Verification items for the finished model (mm, model axes). A direction names the side the tool comes from. Round coordinates to 2 decimals unless told otherwise and drop trailing zeros. Loops run counter-clockwise (first coordinate to the right, second up) from the corner with the lowest first, then second, coordinate; pieces in that order, holes last. Notation, with made-up numbers: M 0,17 L 31,17 A11 cw 31,25 Z; hole C 43.5,42 d4. An arc over 180 degrees is marked long. One line per item, written item: value.
from build123d import *

# Parameters (mm, degrees)
F0_W     = 50
F0_H     = 140
F1_DEPTH = 3
F3_D     = 5
F5_DEPTH = 39.832257


with BuildPart() as f1:
    # F0 (on Top) → F1 (new body)
    with BuildSketch(Plane.XY):
        with Locations((25, 70)):
            Rectangle(F0_W, F0_H)
    extrude(amount=-F1_DEPTH)

    # F3 (through all)
    with Locations(Plane.XY):
        with Locations((30, 86), (30, 62)):
            Hole(F3_D / 2)

    # F4 (on face) → F5 (cut)
    with BuildSketch(Plane.XY):
        with BuildLine():
            ThreePointArc((40.989516, 50), (43.489516, 47.5), (45.989516, 50))
            Line((45.989516, 50), (45.989516, 98))
            ThreePointArc((45.989516, 98), (43.489516, 100.5), (40.989516, 98))
            Line((40.989516, 98), (40.989516, 50))
        make_face()
    extrude(amount=-F5_DEPTH, mode=Mode.SUBTRACT)

    # F6: F1 across plane


with BuildPart() as f1_1:
    add(f1.part)
    add(f1.part.mirror(Plane.YZ))


solid = f1_1.part
(1) Sectioned sample at A-A on x = -30. Enter the section's corners in (y, z).
Completed:
outline: M 0,-3 L 59.5,-3 L 59.5,0 L 0,0 Z; M 64.5,-3 L 83.5,-3 L 83.5,0 L 64.5,0 Z; M 88.5,-3 L 140,-3 L 140,0 L 88.5,0 Z
(2) Sectioned sample at C-C on z = -1.25. Enter the section's corners in (x, y), and give its area (3 significant figures).
Completed:
outline: M -50,0 L 50,0 L 50,140 L -50,140 Z; hole M -45.99,50 A2.5 ccw -40.99,50 L -40.99,98 A2.5 ccw -45.99,98 Z; hole C -30,62 d5; hole C -30,86 d5; hole C 30,62 d5; hole C 30,86 d5; hole M 40.99,50 A2.5 ccw 45.99,50 L 45.99,98 A2.5 ccw 40.99,98 Z
area: 13,400 mm^2
(3) Sectioned sample at B-B on y = 86. Enter the section's corners in (x, z), and give its area (3 significant figures).
Completed:
outline: M -50,-3 L -45.99,-3 L -45.99,0 L -50,0 Z; M -40.99,-3 L -32.5,-3 L -32.5,0 L -40.99,0 Z; M -27.5,-3 L 27.5,-3 L 27.5,0 L -27.5,0 Z; M 32.5,-3 L 40.99,-3 L 40.99,0 L 32.5,0 Z; M 45.99,-3 L 50,-3 L 50,0 L 45.99,0 Z
area: 240 mm^2
(4) Mould release check, pull along X, two halves, no side actions. Record for faces 1 (the face through (1, 0, -1)), 2 (the face through (-50, 69, -1)), 3 (the face through (-43.5, 100.5, -1.5)): +X half, -X half, draft (parallel to the pull), parting line (faces both ways), or undercut.
Completed:
face 1: draft
face 2: -X half
face 3: undercut
(5) Thickness scan on L1, parallel to Y at x = 30, z = -1.7; L2, parallel to X at y = 55.5, z = -0.3; L3, parallel to X at y = 98.5, z = -2.05. Record the ranges inside material, lowest first. Write a range as from..to.
Completed:
L1: y = 0..59.5, 64.5..83.5, 88.5..140
L2: x = -50..-45.99, -40.99..40.99, 45.99..50
L3: x = -50..-45.94, -41.04..41.04, 45.94..50
(6) Tool access check on faces 4 (the face through (50, 69, -1)), 5 (the face through (-43.4, 47.5, -1.5)). Record the directions out of +Z, -Z, +X, -X, +Y, -Y that give a thin tool (end or side, any length) a straight path to the whole face; none if there is none.
Completed:
face 4: +Z, -Z, +X, +Y, -Y
face 5: +Z, -Z
(7) Depth check by flat-ended pin: pin 1 Ø6 at (x, y) = (-39.5, 21.5) entering from +Z. Enter the tip coordinate at first touch or a pass-through.
Completed:
pin 1: stops at z = 0
